from build123d import *

# Parameters (mm, degrees)
BOSS_EXTRUDE1_DEPTH = 4.476
CUT_EXTRUDE1_DEPTH  = 2.413
SKETCH4_R           = 1.65
CUT_EXTRUDE2_DEPTH  = 5.476
CUT_EXTRUDE3_DEPTH  = 3.175
SKETCH6_W           = 16.984037314
SKETCH6_H           = 62.559907231
CUT_EXTRUDE4_DEPTH  = 5.476


with BuildPart() as part:
    # Sketch1 → Boss-Extrude1 (new body)
    with BuildSketch(Plane(origin=(0, 0, 0), x_dir=(1, 0, 0), z_dir=(0, 1, 0))):
        with BuildLine():
            Line((-8.37964191, 28.608687003), (58.93035809, 28.608687003))
            ThreePointArc((58.93035809, 28.608687003), (67.910614211, 24.888943124), (71.63035809, 15.908687003))
            Line((71.63035809, 15.908687003), (71.63035809, -13.301312997))
            ThreePointArc((71.63035809, -13.301312997), (67.910614211, -22.281569118), (58.93035809, -26.001312997))
            Line((58.93035809, -26.001312997), (-8.37964191, -26.001312997))
            ThreePointArc((-8.37964191, -26.001312997), (-12.86976997, -24.141441058), (-14.72964191, -19.651312997))
            Line((-14.72964191, -19.651312997), (-14.72964191, 22.258687003))
            ThreePointArc((-14.72964191, 22.258687003), (-12.86976997, 26.748815063), (-8.37964191, 28.608687003))
        make_face()
    extrude(amount=BOSS_EXTRUDE1_DEPTH)

    # Sketch2 → Cut-Extrude1 (cut)
    with BuildSketch(Plane(origin=(0, 4.476, 0), x_dir=(1, 0, 0), z_dir=(0, 1, 0))):
        Polygon((64.265579696, 19.401187003), (67.565136484, 19.401187003), (69.384674475, 22.552719249), (67.257293816, 25.116187003), (64.265579696, 25.116187003), (62.615801302, 22.258687003), align=None)
        Polygon((69.12572552, -20.413294604), (68.180437233, -17.252044051), (64.970069804, -16.490062445), (62.704990661, -18.889331391), (63.650278947, -22.050581944), (66.860646377, -22.81256355), align=None)
        Polygon((-1.774420304, 22.576187003), (1.525136484, 22.576187003), (3.174914879, 25.433687003), (1.525136484, 28.291187003), (-1.774420304, 28.291187003), (-3.424198698, 25.433687003), align=None)
        Polygon((-1.774420304, -25.683812997), (1.525136484, -25.683812997), (3.174914879, -22.826312997), (1.525136484, -19.968812997), (-1.774420304, -19.968812997), (-3.424198698, -22.826312997), align=None)
    extrude(amount=-CUT_EXTRUDE1_DEPTH, mode=Mode.SUBTRACT)

    # Sketch4 → Cut-Extrude2 (cut, through all)
    with BuildSketch(Plane(origin=(0, 4.476, 0), x_dir=(1, 0, 0), z_dir=(0, 1, 0))):
        with Locations((-0.12464191, 25.433687003)):
            Circle(SKETCH4_R)
        with Locations((-0.12464191, -22.826312997)):
            Circle(SKETCH4_R)
        with Locations((65.91535809, -19.651312997)):
            Circle(SKETCH4_R)
        with Locations((65.91535809, 22.258687003)):
            Circle(SKETCH4_R)
    extrude(amount=-CUT_EXTRUDE2_DEPTH, mode=Mode.SUBTRACT)

    # Sketch5 → Cut-Extrude3 (cut)
    with BuildSketch(Plane(origin=(0, 4.476, 0), x_dir=(1, 0, 0), z_dir=(0, 1, 0))):
        with BuildLine():
            ThreePointArc((18.73485809, 1.303687003), (10.67035809, 9.368187003), (2.60585809, 1.303687003))
            Line((2.60585809, 1.303687003), (18.73485809, 1.303687003))
        make_face()
        with BuildLine():
            Line((18.73485809, 1.303687003), (2.60585809, 1.303687003))
            ThreePointArc((2.60585809, 1.303687003), (10.67035809, -6.760812997), (18.73485809, 1.303687003))
        make_face()
        with BuildLine():
            ThreePointArc((54.29485809, 1.303687003), (46.23035809, 9.368187003), (38.16585809, 1.303687003))
            Line((38.16585809, 1.303687003), (54.29485809, 1.303687003))
        make_face()
        with BuildLine():
            Line((54.29485809, 1.303687003), (38.16585809, 1.303687003))
            ThreePointArc((38.16585809, 1.303687003), (46.23035809, -6.760812997), (54.29485809, 1.303687003))
        make_face()
    extrude(amount=-CUT_EXTRUDE3_DEPTH, mode=Mode.SUBTRACT)

    # Sketch6 → Cut-Extrude4 (cut, through all)
    with BuildSketch(Plane(origin=(0, 4.476, 0), x_dir=(1, 0, 0), z_dir=(0, 1, 0))):
        with Locations((-14.331660567, 1.51751481)):
            Rectangle(SKETCH6_W, SKETCH6_H)
    extrude(amount=-CUT_EXTRUDE4_DEPTH, mode=Mode.SUBTRACT)


solid = part.part
Geometry: final body of the model. Coordinates: model frame, mm. A direction names the side the tool comes from. Give positions to 0.01 mm unless a question says otherwise; leave off trailing zeros. Write each loop counter-clockwise with the first axis right and the second up, starting at its lowest first coordinate (ties: lowest second). Pieces come first, ordered by that corner, then holes. Notation, with made-up numbers: (9, -32) -> (65, -32) arc R21 cw to (65, -11) -> close; hole circle Ø3 at (84, 50). An arc over 180 degrees is marked (long way). Answer as a JSON object with one key per item and string values.
1. Ray query, probe 1 along Z at (x, y) = (46, 3.55); probe 2 along X at (y, z) = (3.8, -5.5); probe 3 along Z at (x, y) = (66, 2.45). Return the intervals inside material, ascending. Write a range as from..to.
Ans:
{"probe 1": "z = -28.61..-9.36, 6.76..26", "probe 2": "x = -5.84..3.78, 17.56..39.34, 53.12..71.63", "probe 3": "z = -26.46..-25.12, -19.4..16.73, 22.61..23.85"}
2. Cut plane C-C on z = 2.5. Output: boundary loops of the cut face in (x, y), and give its area (3 significant figures).
Ans:
{"outline": "(-5.84, 0) -> (71.63, 0) -> (71.63, 4.48) -> (53.34, 4.48) -> (53.34, 1.3) -> (39.12, 1.3) -> (39.12, 4.48) -> (17.78, 4.48) -> (17.78, 1.3) -> (3.56, 1.3) -> (3.56, 4.48) -> (-5.84, 4.48) -> close", "area": "256 mm^2"}
3. Cut plane D-D on x = 11.5. Output: boundary loops of the cut face in (y, z), and give its area (3 significant figures).
Ans:
{"outline": "(0, -28.61) -> (4.48, -28.61) -> (4.48, -9.33) -> (1.3, -9.33) -> (1.3, 6.72) -> (4.48, 6.72) -> (4.48, 26) -> (0, 26) -> close", "area": "193 mm^2"}
4. Cut plane B-B on y = 3.3. Count the separate pieces of the cut face and the enclosed holes in it, and give its area (3 significant figures).
Ans:
{"separate pieces": "1", "enclosed holes": "6", "area": "3,640 mm^2"}
5. Contact query for flat-ended pins moving along their axis: pin 1 (13 mm diameter, centred on x = 10.67, z = -1.3, fed in from +Y); pin 2 (2 mm diameter, centred on x = -0.12, z = 22.83, fed in from -Y); pin 3 (1.9 mm diameter, centred on x = 66.5, y = 3.5, fed in from -Z); pin 4 (1.7 mm diameter, centred on x = 0.5, z = -24, fed in from +Y). Output: stop coordinate, or through.
Ans:
{"pin 1": "stops at y = 1.3", "pin 2": "passes through", "pin 3": "stops at z = -26.75", "pin 4": "stops at y = 2.06"}
6. Mould query, pull axis X, two halves, no side actions, for faces 1 (the flat face through (2.362, 3.286, -26.842)), 2 (the flat face through (33, 0, -2)), 3 (the cylindrical face through (67.8, 2.2, -25)), 4 (the flat face through (-5.84, 2, -1)). Classes: pulls with the +X half, pulls with the -X half, needs draft (parallel to the pull), parting line crosses it, or undercut.
Ans:
{"face 1": "undercut", "face 2": "needs draft", "face 3": "pulls with the +X half", "face 4": "pulls with the -X half"}
7. Cut plane A-A on x = 0. Output: boundary loops of the cut face in (y, z), and give its area (3 significant figures).
Ans:
{"outline": "(0, -28.61) -> (4.48, -28.61) -> (4.48, -28.29) -> (2.06, -28.29) -> (2.06, -27.08) -> (0, -27.08) -> close; (0, -23.79) -> (2.06, -23.79) -> (2.06, -22.58) -> (4.48, -22.58) -> (4.48, 19.97) -> (2.06, 19.97) -> (2.06, 21.18) -> (0, 21.18) -> close; (0, 24.47) -> (2.06, 24.47) -> (2.06, 25.68) -> (4.48, 25.68) -> (4.48, 26) -> (0, 26) -> close", "area": "203 mm^2"}
8. Access query for faces 5 (the flat face through (66, 3, -25.116)), 6 (the cylindrical face through (66.677, 1.046, 21.115)). Directions: +Z, -Z, +X, -X, +Y, -Y. A direction counts if a zero-diameter tool reaches every point of the face in a straight line with its end or side. Return the directions, or none.
Ans:
{"face 5": "+Y", "face 6": "+Y, -Y"}
